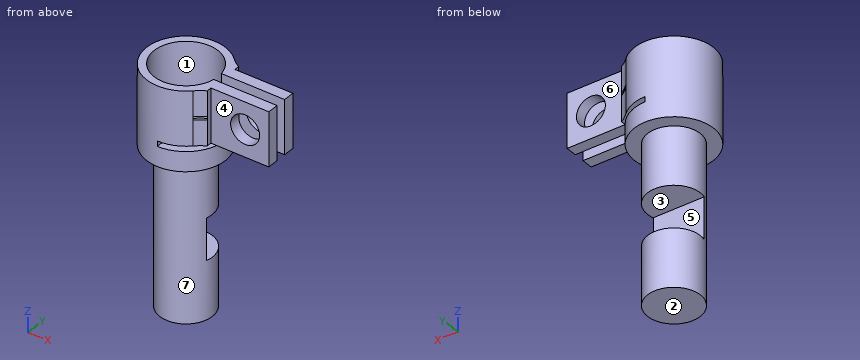
```python
from build123d import *

# Parameters (mm, degrees)
BOSS_EXTRUDE3_DEPTH     = 1.25
SKETCH6_W               = 7.2
SKETCH6_H               = 4.5
CUT_EXTRUDE1_DEPTH      = 0.4
CUT_EXTRUDE2_START      = -4.5
SKETCH7_W               = 8
SKETCH7_H               = 10
CUT_EXTRUDE2_DEPTH      = 0.4
M2_CLEARANCE_HOLE1_D    = 2.2
CUT_EXTRUDE3_DEPTH      = 20.617339269
CUT_EXTRUDE3_DEPTH_BACK = 0.5
SKETCH10_W              = 10
SKETCH10_H              = 3.175
FILLET1_R               = 3.175
CUT_EXTRUDE4_REACH      = 21.847
CUT_EXTRUDE4_END_RADIUS = 3.175
SKETCH12_W              = 4.4
SKETCH12_H              = 4.1


with BuildPart() as part:
    # Sketch3 → Revolve1 (revolve)
    with BuildSketch(Plane(origin=(0, 0, 0), x_dir=(0, 0, -1), z_dir=(1, 0, 0)), mode=Mode.PRIVATE) as revolve1_sk:
        Polygon((18, 0), (18, 2), (6, 2), (6, 3), (0, 3), (0, 2.425), (4.5, 2.425), (4.5, 0), align=None)
    revolve(revolve1_sk.sketch.rotate(Axis((0, 0, 12.785862786), (0, 0, -1)), 90), axis=Axis((0, 0, 12.785862786), (0, 0, -1)))

    # Sketch5 → Boss-Extrude3 (add, symmetric)
    with BuildSketch(Plane(origin=(0, 0, 0), x_dir=(1, 0, 0), z_dir=(0, 1, 0))):
        Polygon((3, 4.5), (7.2, 4.5), (7.2, 0), (3, 0), (2.425, 0), (2.425, 4.5), align=None)
    extrude(amount=BOSS_EXTRUDE3_DEPTH, both=True)

    # Sketch6 → Cut-Extrude1 (cut, symmetric)
    with BuildSketch(Plane(origin=(0, 0, 0), x_dir=(1, 0, 0), z_dir=(0, 1, 0))):
        with Locations((3.6, 2.25)):
            Rectangle(SKETCH6_W, SKETCH6_H)
    extrude(amount=CUT_EXTRUDE1_DEPTH, both=True, mode=Mode.SUBTRACT)

    # Sketch7 → Cut-Extrude2 (cut)
    with BuildSketch(Plane.XY.offset(CUT_EXTRUDE2_START)):
        with Locations((4, 0)):
            Rectangle(SKETCH7_W, SKETCH7_H)
    extrude(amount=CUT_EXTRUDE2_DEPTH, mode=Mode.SUBTRACT)

    # M2 Clearance Hole1 (through all)
    with Locations(Plane(origin=(0, 1.25, 0), x_dir=(1, 0, 0), z_dir=(0, 1, 0))):
        with Locations((5.4, 2.05)):
            Hole(M2_CLEARANCE_HOLE1_D / 2)

    # Sketch10 → Cut-Extrude3 (cut, two sides: drawn at the far end of the back side and taken through both)
    with BuildSketch(Plane(origin=(0, 0, 0), x_dir=(1, 0, 0), z_dir=(0, 1, 0)).offset(-CUT_EXTRUDE3_DEPTH_BACK)):
        with Locations((0, 12)):
            Rectangle(SKETCH10_W, SKETCH10_H)
    extrude(amount=CUT_EXTRUDE3_DEPTH + CUT_EXTRUDE3_DEPTH_BACK, mode=Mode.SUBTRACT)

    # Fillet1
    fillet1_edges = [part.edges().sort_by_distance(p)[0] for p in [
        (2.727178029, -1.25, -2.05),
        (2.727178029, 1.25, -2.05),
    ]]
    fillet(fillet1_edges, radius=FILLET1_R)

    # Cut-Extrude4: up to this cylinder (the profile starts outside it)
    cut_extrude4_end = Plane(origin=(4.306971093, 4.425, -2.05), z_dir=(0, 0, 1)) * Cylinder(CUT_EXTRUDE4_END_RADIUS, 51.044, mode=Mode.PRIVATE)
    # Sketch12 → Cut-Extrude4 (cut, up to the surface)
    with BuildSketch(Plane(origin=(0, 1.25, 0), x_dir=(1, 0, 0), z_dir=(0, 1, 0)), mode=Mode.PRIVATE) as cut_extrude4_sk1:
        with Locations((5, 2.05)):
            Rectangle(SKETCH12_W, SKETCH12_H)
    cut_extrude4_tool1 = extrude(cut_extrude4_sk1.sketch, amount=CUT_EXTRUDE4_REACH, mode=Mode.PRIVATE) - cut_extrude4_end
    cut_extrude4 = cut_extrude4_tool1.solids().sort_by_distance((5, 1.25, -2.05))[0] + cut_extrude4_tool1.solids().sort_by_distance((5, 1.25, -2.05))[1]
    add(cut_extrude4, mode=Mode.SUBTRACT)

    # Mirror1: Cut-Extrude4 across plane
    add(cut_extrude4.mirror(Plane.ZX), mode=Mode.SUBTRACT)


solid = part.part
```
Could you check a few things on this model? Use its own coordinates, in mm. Face numbers are marked on the shaded views. A direction names the side the tool comes from. Round coordinates to 2 decimals unless told otherwise and drop trailing zeros. Write each loop counter-clockwise with the first axis right and the second up, starting at its lowest first coordinate (ties: lowest second). Pieces come first, ordered by that corner, then holes.
(1) If I drill on probe 1 along Z at (x, y) = (5.4, 0.65); probe 2 along Y at (x, z) = (0, -2.85) (3 decimals); probe 3 along Z at (x, y) = (1, 2.25), over which ranges is the centre line in solid material (lowest first)?
Findings below:
probe 1: z = -4.1 to -3.15, -0.95 to 0
probe 2: y = -3 to -2.425, 2.425 to 3
probe 3: z = -6 to -4.5, -4.1 to 0
(2) For pin 1 (1.2 mm diameter, centred on x = 5.5, z = -1.5, fed in from +Y); pin 2 (3.5 mm diameter, centred on x = 5, z = -2, fed in from -Y); pin 3 (1.3 mm diameter, centred on x = 5, y = 1, fed in from -Z), each with a flat end and sliding along its axis, tell me the tip position at first contact or that it passes through.
Findings below:
pin 1: stops at y = 1.25
pin 2: stops at y = -1.25
pin 3: stops at z = -4.1
(3) Suppose I cut it at C-C on y = 0. Write out the boundary of the cut face in (x, z) (1 decimal).
Findings below:
outline: (-3, -6) - (-2, -6) - (-2, -10.4) - (2, -10.4) - (2, -6) - (3, -6) - (3, -4.5) - (-2.4, -4.5) - (-2.4, 0) - (-3, 0) - close; (-2, -18) - (2, -18) - (2, -13.6) - (-2, -13.6) - close
(4) Suppose I cut it at B-B on x = 3.75. Write out the boundary of the cut face in (y, z).
Findings below:
outline: (-1.25, -4.1) - (-0.4, -4.1) - (-0.4, 0) - (-1.25, 0) - close; (0.4, -4.1) - (1.25, -4.1) - (1.25, 0) - (0.4, 0) - close
(5) Which directions (+Z, -Z, +X, -X, +Y, -Y) give clear straight access to the entire face, cutting with the end or side of a thin tool? Please do the marked faces 4, 5, 6 and 7.
Findings below:
face 4: +Z, -Z, +X, -Y
face 5: +X, -X, +Y
face 6: +Z, -Z, +X, +Y
face 7: -Z
(6) Thinking about a two-plate mould opening in Z: for the marked faces 1, 2 and 3, which applies, +Z half, -Z half, draft (parallel to the pull), parting line (faces both ways), or undercut?
Findings below:
face 1: draft
face 2: -Z half
face 3: undercut
(7) Suppose I cut it at D-D on y = 1. Write out the boundary of the cut face in (x, z).
Findings below:
outline: (-2.83, -6) - (-1.73, -6) - (-1.73, -10.41) - (1.73, -10.41) - (1.73, -6) - (2.83, -6) - (2.83, -4.5) - (-2.21, -4.5) - (-2.21, 0) - (-2.83, 0) - close; (-1.73, -18) - (1.73, -18) - (1.73, -13.59) - (-1.73, -13.59) - close; (2.21, -4.1) - (7.2, -4.1) - (7.2, 0) - (2.21, 0) - close; hole circle Ø2.2 at (5.4, -2.05)
(8) Suppose I cut it at A-A on x = 5.4. Write out the boundary of the cut face in (y, z), and give its area (3 significant figures).
Findings below:
outline: (-1.25, -4.1) - (-0.4, -4.1) - (-0.4, -3.15) - (-1.25, -3.15) - close; (-1.25, -0.95) - (-0.4, -0.95) - (-0.4, 0) - (-1.25, 0) - close; (0.4, -4.1) - (1.25, -4.1) - (1.25, -3.15) - (0.4, -3.15) - close; (0.4, -0.95) - (1.25, -0.95) - (1.25, 0) - (0.4, 0) - close
area: 3.23 mm2
